Could you check a few things on this model? Use its own coordinates, in mm. A direction names the side the tool comes from. Give positions to 0.01 mm unless a question says otherwise; leave off trailing zeros. Loops run counter-clockwise (first coordinate to the right, second up) from the corner with the lowest first, then second, coordinate; pieces in that order, holes last. Notation, with made-up numbers: (2, 76) - (21, 76) arc R29 cw to (21, 108) - close; hole circle Ø4 at (76, 59.5). An arc over 180 degrees is marked (long way). Write each question's results on one line, items separated by ' | '. Start each with the question number.
1) If I drill on probe 1 along X at (y, z) = (0, -1.5); probe 2 along Y at (x, z) = (-17.75, -2); probe 3 along Z at (x, y) = (-19, 1.5), over which ranges is the centre line in solid material (lowest first)? Write a range as [from, to].
2) I want a section at C-C, the plane x = -3.5. Write out the boundary of the cut face in (y, z), and give its area (3 significant figures).
3) On a 3-axis mill with a long thin cutter (end or side, diameter ignored), from which of +Z, -Z, +X, -X, +Y, -Y can I reach the whole of each face in a straight line? I mean faces 1 (the face through (-8.1, -0.1, -2.5)), 2 (the face through (-19, 0.5, 1)), 3 (the face through (-19.6, 1, -1)). Say none if no direction works.
4) I'm going to push flat-ended pins straight in: pin 1 (1.4 mm diameter, centred on x = -19, y = 1, fed in from +Z); pin 2 (1.5 mm diameter, centred on x = -6, z = 3, fed in from -Y); pin 3 (1.4 mm diameter, centred on x = -18.5, z = -1, fed in from +Y). Where does each tip first touch, or does it pass through?
5) I want a section at A-A, the plane z = 0. Write out the boundary of the cut face in (x, y), and give its area (3 significant figures).
6) If we mould it in two halves opening along Z, with no side actions, what happens to faces 4 (the face through (0, 0, 0)), 5 (the face through (-16.651, 2.535, -0.563)), 6 (the face through (-19, 0, -2.25))? For each: +Z half, -Z half, draft (parallel to the pull), parting line (faces both ways), or undercut.
from build123d import *

# Parameters (mm, degrees)
SKETCH_2_W          = 1
SKETCH_2_H          = 1.75
SKETCH_2_W_2        = 1.75
SKETCH_2_H_2        = 1
CUT_EXTRUDE_1_DEPTH = 2


with BuildPart() as part:
    # Эскиз1 → Повернуть1 (revolve)
    with BuildSketch(Plane.XY, mode=Mode.PRIVATE) as revolve_1_sk:
        Polygon((-19.6, 0), (-19.6, 4.5), (-16.5, 2.5), (0, 2.5), (0, 0), align=None)
    revolve(revolve_1_sk.sketch.rotate(Axis((-51.630571285, 0, 0), (1, 0, 0)), 90), axis=Axis((-51.630571285, 0, 0), (1, 0, 0)))

    # Эскиз2 → Вырез-Вытянуть1 (cut)
    with BuildSketch(Plane.ZY.offset(19.6)):
        with Locations((0, 1.375)):
            Rectangle(SKETCH_2_W, SKETCH_2_H)
        with Locations((1.375, 0)):
            Rectangle(SKETCH_2_W_2, SKETCH_2_H_2)
        with Locations((0, -1.375)):
            Rectangle(SKETCH_2_W, SKETCH_2_H)
        with Locations((-1.375, 0)):
            Rectangle(SKETCH_2_W_2, SKETCH_2_H_2)
        Rectangle(SKETCH_2_W, SKETCH_2_H_2)
    extrude(amount=-CUT_EXTRUDE_1_DEPTH, mode=Mode.SUBTRACT)


solid = part.part
Answers:
1) probe 1: x = [-17.6, 0] | probe 2: y = [-2.63, -0.5], [0.5, 2.63] | probe 3: z = [-3.83, -0.5], [0.5, 3.83]
2) outline: circle Ø5 at (0, 0) | area: 19.6 mm2
3) face 1: +X | face 2: -X | face 3: +Z, -Z, -X, +Y, -Y
4) pin 1: stops at z = 4.45 | pin 2: stops at y = -1.09 | pin 3: stops at y = 4.15
5) outline: (-19.6, -4.5) - (-16.5, -2.5) - (0, -2.5) - (0, 2.5) - (-16.5, 2.5) - (-19.6, 4.5) - (-19.6, 2.25) - (-17.6, 2.25) - (-17.6, -2.25) - (-19.6, -2.25) - close | area: 95.2 mm2
6) face 4: draft | face 5: parting line | face 6: undercut
